Part model, mm, in its own coordinate system. A direction names the side the tool comes from. Coordinates: 2 decimals unless noted, no trailing zeros. Write each loop counter-clockwise with the first axis right and the second up, starting at its lowest first coordinate (ties: lowest second). Pieces come first, ordered by that corner, then holes. Notation, with made-up numbers: (41, 43) -> (61, 43) arc R16 ccw to (61, 50) -> close; hole circle Ø6 at (75.5, 32.5). An arc over 180 degrees is marked (long way). Write item = value, one per line. Start each with the question number.
Q1. Band-saw the part on B-B, the plane z = 1. List the corners of the cut face in (x, y).
Q2. Probe line 1 (X direction, y = 3.3, z = 0); line 2 (X direction, y = 3.9, z = -7); line 3 (X direction, y = 4.7, z = 0). List the from-to ranges inside material, lowest first.
Q3. Band-saw the part on C-C, the plane z = -5.5. List the corners of the cut face in (x, y), plus the area to 3 significant figures.
Q4. Pin check, flat tips, straight feed: P1, Ø10, axis at x = 7, z = -6.5, coming from the -Y side; P2, Ø5, axis at x = 0, z = 0, coming from the +Y side; P3, Ø6, axis at x = -6, z = -6, coming from the +Y side; P4, Ø2.5, axis at x = 0, z = 0, coming from the +Y side. Stop position of each tip, or through.
Q5. Pull direction X, two halves, no side cores. Call faces 1 (the cylindrical face through (-3.04, 1.23, 3.32)), 2 (the flat face through (5, 2.5, 0)), 3 (the cylindrical face through (-8.475, 3.514, -3.016)): released by +X, released by -X, zero draft, split by the parting line, or undercut.
Q6. Band-saw the part on D-D, the plane y = 1.45. List the corners of the cut face in (x, z).
Q7. Tool access for faces 4 (the flat face through (-3, 5, 1)), 5 (the cylindrical face through (-0.9, 4.51, -2.86)), 6 (the cylindrical face through (2.685, 1.521, 0.596)): list every direction of +Z, -Z, +X, -X, +Y, -Y with a clear straight run to the whole face (end or side of a thin tool).
Q8. Band-saw the part on A-A, the plane x = 6.5. List the corners of the cut face in (y, z).
from build123d import *

# Parameters (mm, degrees)
ESQUISSE2_R                  = 0.5
ENL_V_MAT_EXTRU_1_DEPTH      = 10
R_P_TITION_CIRCULAIRE1_COUNT = 3
R_P_TITION_CIRCULAIRE1_ANGLE = 40


with BuildPart() as part:
    # Esquisse1 → Révolution1 (revolve)
    with BuildSketch(Plane.XY, mode=Mode.PRIVATE) as r_volution1_sk:
        Polygon((2.75, 0), (2.75, 3), (1.5, 3), (1.5, 4), (3, 4), (3, 5), (3.75, 5), (3.75, 4.5), (12, 4.5), (12, 2.5), (4.5, 2.5), (4.5, 0), align=None)
    revolve(r_volution1_sk.sketch.rotate(Axis((0, 0, 0), (0, 1, 0)), 90), axis=Axis((0, 0, 0), (0, 1, 0)))

    # Esquisse2 → Enlèv. mat.-Extru.1 (cut)
    with BuildSketch(Plane(origin=(0, 4.5, 0), x_dir=(1, 0, 0), z_dir=(0, 1, 0))):
        with Locations(Location((0, 10, 0), (0, 0, 270))):
            Circle(ESQUISSE2_R)
        with Locations(Location((8.5, 0, 0), (0, 0, 270))):
            Circle(ESQUISSE2_R)
        with Locations(Location((0, 7, 0), (0, 0, 270))):
            Circle(ESQUISSE2_R)
        with Locations(Location((0, -7, 0), (0, 0, 90))):
            Circle(ESQUISSE2_R)
        with Locations(Location((0, -10, 0), (0, 0, 90))):
            Circle(ESQUISSE2_R)
        with Locations(Location((-8.5, 0, 0), (0, 0, 90))):
            Circle(ESQUISSE2_R)
    enl_v_mat_extru_1 = extrude(amount=-ENL_V_MAT_EXTRU_1_DEPTH, mode=Mode.SUBTRACT)

    # Répétition circulaire1: Enlèv. mat.-Extru.1 ×3 about axis
    r_p_tition_circulaire1_axis = Axis((0, 0, 0), (0, -1, 0))
    for i in range(1, R_P_TITION_CIRCULAIRE1_COUNT):
        add(enl_v_mat_extru_1.rotate(r_p_tition_circulaire1_axis, i * R_P_TITION_CIRCULAIRE1_ANGLE / (R_P_TITION_CIRCULAIRE1_COUNT - 1)), mode=Mode.SUBTRACT)


solid = part.part
Ans:
q1.outline = (-11.96, 2.5) -> (-4.39, 2.5) -> (-4.39, 0) -> (-2.56, 0) -> (-2.56, 3) -> (-1.12, 3) -> (-1.12, 4) -> (-2.83, 4) -> (-2.83, 5) -> (-3.61, 5) -> (-3.61, 4.5) -> (-11.96, 4.5) -> close; (1.12, 3) -> (2.56, 3) -> (2.56, 0) -> (4.39, 0) -> (4.39, 2.5) -> (11.96, 2.5) -> (11.96, 4.5) -> (3.61, 4.5) -> (3.61, 5) -> (2.83, 5) -> (2.83, 4) -> (1.12, 4) -> close
q2.line_1 = -12 to -9, -8 to -1.5, 1.5 to 8, 9 to 12
q2.line_2 = -9.75 to -0.5, 0.5 to 2.13, 2.66 to 9.75
q2.line_3 = -3.75 to -3, 3 to 3.75
q3.outline = (-10.67, 2.5) -> (-7.01, 2.5) -> (-7.01, 4.5) -> (-10.67, 4.5) -> close; (-6.01, 2.5) -> (4.02, 2.5) -> (4.02, 4.5) -> (-6.01, 4.5) -> close; (4.98, 2.5) -> (10.67, 2.5) -> (10.67, 4.5) -> (4.98, 4.5) -> close
q3.area = 38.7 mm2
q4.P1 = 2.5
q4.P2 = 4
q4.P3 = 4.5
q4.P4 = through
q5.face_1 = split by the parting line
q5.face_2 = zero draft
q5.face_3 = undercut
q6.outline = circle Ø9 at (0, 0); hole circle Ø5.5 at (0, 0)
q7.face_4 = +Z, -Z, +X, -X, +Y
q7.face_5 = +Y
q7.face_6 = -Y
q8.outline = (2.5, -10.09) -> (4.5, -10.09) -> (4.5, -8.16) -> (2.5, -8.16) -> close; (2.5, -7.17) -> (4.5, -7.17) -> (4.5, 4.96) -> (2.5, 4.96) -> close; (2.5, 5.96) -> (4.5, 5.96) -> (4.5, 10.09) -> (2.5, 10.09) -> close
